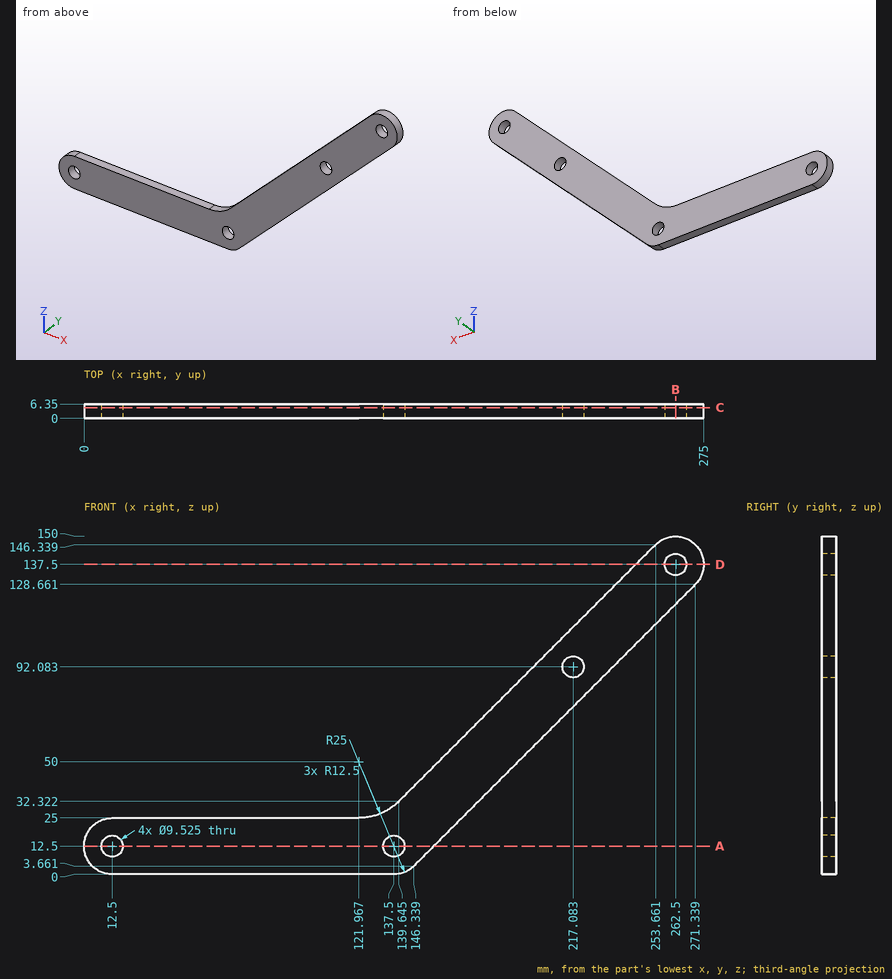
Part print with two shaded views. Sizes in mm from the minimum x, y, z corner. Coordinates: 2 decimals unless noted, no trailing zeros. Write each loop counter-clockwise with the first axis right and the second up, starting at its lowest first coordinate (ties: lowest second). Pieces come first, ordered by that corner, then holes. Notation, with made-up numbers: (57, -24.75) - (97, -24.75) arc R15 cw to (97, -18.75) - close; hole circle Ø6 at (-34.5, -31). An arc over 180 degrees is marked (long way). Use a Markdown table: item, result. Add a question column.
Item 1: Band-saw the part on B-B, the plane x = 262.5. Write the cut outline in (y, z).
Item 2: Band-saw the part on C-C, the plane y = 4.75. Write the cut outline in (x, z) (1 decimal), and give its area (3 significant figures).
Item 3: Drill centre lines: line 1 along X through (y, z) = (1.5, 12.5); line 2 along X through (y, z) = (3.75, 9.5) (1 decimal); line 3 along Z through (x, y) = (115, 3.25). Where is each one in solid material? Low to high.
Item 4: Drop flat-ended pins along their axis: pin 1 (1.9 mm diameter, centred on x = 90, y = 2.5, fed in from +Z); pin 2 (7.5 mm diameter, centred on x = 137.5, z = 12.5, fed in from -Y); pin 3 (1.5 mm diameter, centred on y = 3.5, z = 34, fed in from +X); pin 4 (2 mm diameter, centred on x = 195, y = 4.5, fed in from -Z). Give the stop position or say it passes through.
Item 5: Band-saw the part on A-A, the plane z = 12.5. Write the cut outline in (x, y).
Item 6: Band-saw the part on D-D, the plane z = 137.5. Write the cut outline in (x, y).
A:
| question | item | result |
|---|---|---|
| 1 | outline | (0, 119.82) - (6.35, 119.82) - (6.35, 132.74) - (0, 132.74) - close; (0, 142.26) - (6.35, 142.26) - (6.35, 150) - (0, 150) - close |
| 2 | outline | (12.5, 0) - (137.5, 0) arc R12.5 ccw to (146.3, 3.7) - (271.3, 128.7) arc R12.5 ccw to (253.7, 146.3) - (139.6, 32.3) arc R25 cw to (122, 25) - (12.5, 25) arc R12.5 ccw to start; hole circle Ø9.5 at (12.5, 12.5); hole circle Ø9.5 at (137.5, 12.5); hole circle Ø9.5 at (217.1, 92.1); hole circle Ø9.5 at (262.5, 137.5) |
| 2 | area | 7,760 mm² |
| 3 | line 1 | x = 0 to 7.74, 17.26 to 132.74, 142.26 to 155.18 |
| 3 | line 2 | x = 0.4 to 8.8, 16.2 to 133.8, 141.2 to 152.2 |
| 3 | line 3 | z = 0 to 25 |
| 4 | pin 1 | stops at z = 25 |
| 4 | pin 2 | passes through |
| 4 | pin 3 | stops at x = 177.43 |
| 4 | pin 4 | stops at z = 51.32 |
| 5 | outline | (0, 0) - (7.74, 0) - (7.74, 6.35) - (0, 6.35) - close; (17.26, 0) - (132.74, 0) - (132.74, 6.35) - (17.26, 6.35) - close; (142.26, 0) - (155.18, 0) - (155.18, 6.35) - (142.26, 6.35) - close |
| 6 | outline | (244.82, 0) - (257.74, 0) - (257.74, 6.35) - (244.82, 6.35) - close; (267.26, 0) - (275, 0) - (275, 6.35) - (267.26, 6.35) - close |
